Source: CAD feature listing. Evaluate the final solid. Frame: model axes, mm. A direction names the side the tool comes from. Round coordinates to 2 decimals unless told otherwise and drop trailing zeros. Order: outer loops, then holes, each group sorted by start corner. A loop starts at its lowest first (then second) coordinate and runs counter-clockwise, first axis right, second up.
```python
from build123d import *

# Parameters (mm, degrees)
SKETCH1_R           = 4.5
BOSS_EXTRUDE1_DEPTH = 7
SKETCH2_W           = 25
SKETCH2_H           = 20
CUT_EXTRUDE1_DEPTH  = 3.5
SKETCH3_R           = 1.35
CUT_EXTRUDE2_DEPTH  = 14
FILLET2_R           = 1.2
SKETCH4_R           = 7.5
CUT_EXTRUDE3_DEPTH  = 1
SKETCH5_R           = 6.5
CUT_EXTRUDE4_DEPTH  = 4
FILLET3_R           = 15
SKETCH6_W           = 5
SKETCH6_H           = 5
BOSS_EXTRUDE2_DEPTH = 7
FILLET4_R           = 2
SKETCH7_W           = 110.688595786
SKETCH7_H           = 55.300338959
CUT_EXTRUDE5_DEPTH  = 7


with BuildPart() as part:
    # Sketch1 → Boss-Extrude1 (new body)
    with BuildSketch(Plane(origin=(0, 0, 0), x_dir=(1, 0, 0), z_dir=(0, 1, 0))):
        Polygon((0, 0), (55, 0), (55, -4), (85, -4), (85, 0), (85, 20), (0, 20), align=None)
        with Locations(Location((70, 5, 0), (0, 0, 270))):
            Circle(SKETCH1_R, mode=Mode.SUBTRACT)
    extrude(amount=BOSS_EXTRUDE1_DEPTH)

    # Sketch2 → Cut-Extrude1 (cut)
    with BuildSketch(Plane.XZ):
        with Locations((12.5, -10)):
            Rectangle(SKETCH2_W, SKETCH2_H)
    extrude(amount=-CUT_EXTRUDE1_DEPTH, mode=Mode.SUBTRACT)

    # Sketch3 → Cut-Extrude2 (cut)
    with BuildSketch(Plane.XZ.offset(-3.5)):
        with Locations(Location((5, -4, 0), (0, 0, 270))):
            Circle(SKETCH3_R)
        with Locations(Location((20, -4, 0), (0, 0, 270))):
            Circle(SKETCH3_R)
        with Locations(Location((20, -16, 0), (0, 0, 270))):
            Circle(SKETCH3_R)
        with Locations(Location((5, -16, 0), (0, 0, 270))):
            Circle(SKETCH3_R)
    extrude(amount=-CUT_EXTRUDE2_DEPTH, mode=Mode.SUBTRACT)

    # Fillet2
    fillet2_edges = [part.edges().sort_by_distance(p)[0] for p in [
        (55, 3.5, 4),
        (55, 3.5, 0),
    ]]
    fillet(fillet2_edges, radius=FILLET2_R)

    # Sketch4 → Cut-Extrude3 (cut)
    with BuildSketch(Plane(origin=(0, 7, 0), x_dir=(1, 0, 0), z_dir=(0, 1, 0))):
        with Locations(Location((70, 5, 0), (0, 0, 270))):
            Circle(SKETCH4_R)
    extrude(amount=-CUT_EXTRUDE3_DEPTH, mode=Mode.SUBTRACT)

    # Sketch5 → Cut-Extrude4 (cut)
    with BuildSketch(Plane(origin=(0, 6, 0), x_dir=(1, 0, 0), z_dir=(0, 1, 0))):
        with Locations(Location((70, 5, 0), (0, 0, 270))):
            Circle(SKETCH5_R)
    extrude(amount=-CUT_EXTRUDE4_DEPTH, mode=Mode.SUBTRACT)

    # Fillet3
    fillet3_edges = [part.edges().sort_by_distance(p)[0] for p in [
        (85, 3.5, 4),
    ]]
    fillet(fillet3_edges, radius=FILLET3_R)

    # Sketch6 → Boss-Extrude2 (add)
    with BuildSketch(Plane(origin=(0, 7, 0), x_dir=(1, 0, 0), z_dir=(0, 1, 0))):
        with Locations((82.5, 22.5)):
            Rectangle(SKETCH6_W, SKETCH6_H)
    extrude(amount=-BOSS_EXTRUDE2_DEPTH)

    # Fillet4
    fillet4_edges = [part.edges().sort_by_distance(p)[0] for p in [
        (80, 3.5, -25),
        (80, 3.5, -20),
        (85, 3.5, -25),
    ]]
    fillet(fillet4_edges, radius=FILLET4_R)

    # Mirror1: part across plane


with BuildPart() as part_1:
    add(part.part)
    add(part.part.mirror(Plane(origin=(0, 0, 0), x_dir=(0, 0, 1), z_dir=(0, -1, 0))))

    # Sketch7 → Cut-Extrude5 (cut)
    with BuildSketch(Plane(origin=(0, 7, 0), x_dir=(1, 0, 0), z_dir=(0, 1, 0))):
        with Locations((37.884311931, 10.917741369)):
            Rectangle(SKETCH7_W, SKETCH7_H)
    extrude(amount=-CUT_EXTRUDE5_DEPTH, mode=Mode.SUBTRACT)


solid = part_1.part
```
1. First-contact query: pin 1 (2 mm diameter, centred on x = 34.5, y = -2, fed in from +Z); pin 2 (1 mm diameter, centred on y = -1.5, z = -13.5, fed in from -X); pin 3 (4 mm diameter, centred on y = -3.5, z = -5.5, fed in from +X). Flat tips, straight axial feed; report the tip coordinate or a pass-through.
2. Access query for faces 5 (the face through (33, -4, 0)), 6 (the face through (25, -2, -10)), 7 (the face through (71.54, -2, -9.42)), 8 (the face through (48, -3, -20)), 9 (the face through (63, -3, 4)). Directions: +Z, -Z, +X, -X, +Y, -Y. A direction counts if a zero-diameter tool reaches every point of the face in a straight line with its end or side. Return the directions, or none.
3. Pull-direction query (X, two-part tool) for faces 1 (the face through (12, -3.5, -10)), 2 (the face through (5.912, -5.226, -15.005)), 3 (the face through (55, -3, 2)), 4 (the face through (63.655, -4.028, -6.409)); classes: released by +X, released by -X, zero draft, split by the parting line, or undercut.
4. Line query: line 1 along Z through (x, y) = (70, -1.1); line 2 along X through (y, z) = (-6, -17); line 3 along Y through (x, z) = (19.5, -0.5). Output: solid intervals per line, ascending.
5. Section A-A on z = -16. Return loops of the section in (x, y).
6. Section D-D on z = -4. Return loops of the section in (x, y), plus the area to 3 significant figures.
7. Section C-C on y = -4.75. Return loops of the section in (x, z).
8. Section B-B on x = 5. Return loops of the section in (y, z).
Result:
1. pin 1: stops at z = 0
1. pin 2: stops at x = 25
1. pin 3: stops at x = 84.59
2. face 5: +Z, -X, +Y, -Y
2. face 6: +Z, -Z, -X, +Y
2. face 7: -Y
2. face 8: -Z, -X, +Y, -Y
2. face 9: +Z, +X, -X, +Y, -Y
3. face 1: zero draft
3. face 2: undercut
3. face 3: released by -X
3. face 4: undercut
4. line 1: z = -20 to -9.5, -0.5 to 4
4. line 2: x = 0 to 4.09, 5.91 to 19.09, 20.91 to 85
4. line 3: y = -7 to -3.5
5. outline: (0, -7) - (3.65, -7) - (3.65, -3.5) - (0, -3.5) - close; (6.35, -7) - (18.65, -7) - (18.65, -3.5) - (6.35, -3.5) - close; (21.35, -7) - (85, -7) - (85, 0) - (25, 0) - (25, -3.5) - (21.35, -3.5) - close
6. outline: (0, -7) - (3.65, -7) - (3.65, -3.5) - (0, -3.5) - close; (6.35, -7) - (18.65, -7) - (18.65, -3.5) - (6.35, -3.5) - close; (21.35, -7) - (62.57, -7) - (62.57, -6) - (63.58, -6) - (63.58, -2) - (65.61, -2) - (65.61, 0) - (25, 0) - (25, -3.5) - (21.35, -3.5) - close; (74.39, -2) - (76.42, -2) - (76.42, -6) - (77.43, -6) - (77.43, -7) - (83.27, -7) - (83.27, 0) - (74.39, 0) - close
6. area: 393 mm2
7. outline: (0, -20) - (78, -20) arc R2 cw to (80, -22) - (80, -23) arc R2 ccw to (82, -25) - (83, -25) arc R2 ccw to (85, -23) - (85, -11) arc R15 ccw to (70, 4) - (56.2, 4) arc R1.2 ccw to (55, 2.8) - (55, 1.2) arc R1.2 cw to (53.8, 0) - (0, 0) - close; hole circle Ø2.7 at (5, -16); hole circle Ø2.7 at (5, -4); hole circle Ø2.7 at (20, -16); hole circle Ø2.7 at (20, -4); hole circle Ø13 at (70, -5)
8. outline: (-7, -20) - (-3.5, -20) - (-3.5, -17.35) - (-7, -17.35) - close; (-7, -14.65) - (-3.5, -14.65) - (-3.5, -5.35) - (-7, -5.35) - close; (-7, -2.65) - (-3.5, -2.65) - (-3.5, 0) - (-7, 0) - close
